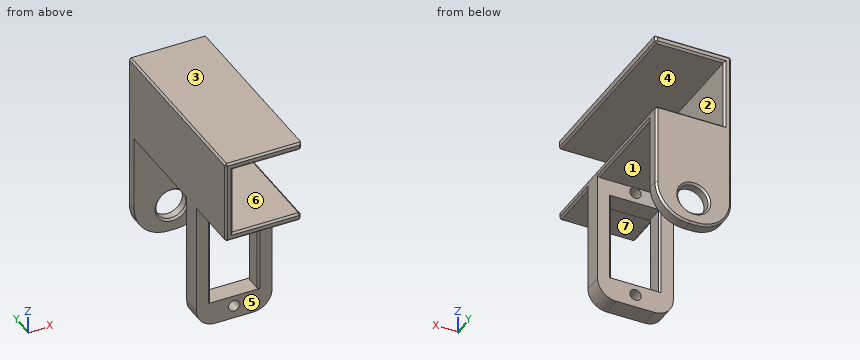
from build123d import *

# Parameters (mm, degrees)
SKETCH1_W           = 20
SKETCH1_H           = 50
BOSS_EXTRUDE1_DEPTH = 2
BOSS_EXTRUDE2_DEPTH = 50
SKETCH3_R           = 4
BOSS_EXTRUDE3_DEPTH = 3
SKETCH4_W           = 12.6
SKETCH4_H           = 23.6
BOSS_EXTRUDE4_DEPTH = 5
CHAMFER1_SIZE       = 0.5
CHAMFER2_SIZE       = 0.5
SKETCH5_R           = 1.5
CUT_EXTRUDE1_DEPTH  = 5


with BuildPart() as part:
    # Sketch1 → Boss-Extrude1 (new body)
    with BuildSketch(Plane.XY):
        with Locations((0, 25)):
            Rectangle(SKETCH1_W, SKETCH1_H)
    extrude(amount=BOSS_EXTRUDE1_DEPTH)

    # Sketch2 → Boss-Extrude2 (add)
    with BuildSketch(Plane.XZ):
        Polygon((-10, 2), (-10, 22.1), (10.1, 22.1), (10.1, 20.1), (-8, 20.1), (-8, 2), align=None)
    extrude(amount=-BOSS_EXTRUDE2_DEPTH)

    # Sketch3 → Boss-Extrude3 (add)
    with BuildSketch(Plane(origin=(0, 50, 0), x_dir=(1, 0, 0), z_dir=(0, 1, 0))):
        with BuildLine():
            Line((1, 28.638755942), (-1, 28.638755942))
            ThreePointArc((-1, 28.638755942), (-7.363961031, 26.002716972), (-10, 19.638755942))
            Line((-10, 19.638755942), (-10, 0))
            Line((-10, 0), (10, 0))
            Line((10, 0), (10, 19.638755942))
            ThreePointArc((10, 19.638755942), (7.363961031, 26.002716972), (1, 28.638755942))
        make_face()
        with Locations(Location((0, 21.5, 0), (0, 0, 270))):
            Circle(SKETCH3_R, mode=Mode.SUBTRACT)
    extrude(amount=-BOSS_EXTRUDE3_DEPTH)

    # Sketch4 → Boss-Extrude4 (add)
    with BuildSketch(Plane(origin=(0, 20, 0), x_dir=(-1, 0, 0), z_dir=(0, -1, 0))):
        with BuildLine():
            Line((-10, 0), (10, 0))
            Line((10, 0), (10, 29))
            ThreePointArc((10, 29), (8.535533906, 32.535533906), (5, 34))
            Line((5, 34), (-5, 34))
            ThreePointArc((-5, 34), (-8.535533906, 32.535533906), (-10, 29))
            Line((-10, 29), (-10, 0))
        make_face()
        with Locations((0, 16)):
            Rectangle(SKETCH4_W, SKETCH4_H, mode=Mode.SUBTRACT)
    extrude(amount=BOSS_EXTRUDE4_DEPTH)

    # Chamfer1
    chamfer1_edges = [part.edges().sort_by_distance(p)[0] for p in [
        (1, 0, 2),
        (-10, 25, 22.1),
        (10.1, 25, 20.1),
        (-8, 0, 11.05),
        (1.05, 0, 20.1),
        (10.1, 0, 21.1),
        (0.05, 0, 22.1),
        (0.05, 50, 22.1),
        (10.1, 50, 21.1),
        (1.05, 50, 20.1),
        (-8, 50, 11.05),
        (-10, 33.5, 0),
        (0, 50, -25.5),
        (0, 50, -28.638755942),
        (-7.363961031, 50, -26.002716972),
        (7.363961031, 50, -26.002716972),
        (10, 25, 2),
        (0, 0, 0),
        (-10, 7.5, 0),
        (10, 33.5, 0),
        (6.3, 20, -16),
        (-6.3, 20, -16),
        (6.3, 15, -16),
        (10, 7.5, 0),
        (-6.3, 15, -16),
        (1, 50, 2),
        (10, 0, 1),
        (-10, 0, 11.05),
        (-10, 50, 1.230622029),
        (10, 50, -8.819377971),
    ]]
    chamfer(chamfer1_edges, length=CHAMFER1_SIZE)

    # Chamfer2
    chamfer2_edges = [part.edges().sort_by_distance(p)[0] for p in [
        (0, 47, -25.5),
    ]]
    chamfer(chamfer2_edges, length=CHAMFER2_SIZE)

    # Sketch5 → Cut-Extrude1 (cut)
    with BuildSketch(Plane(origin=(0, 20, 0), x_dir=(1, 0, 0), z_dir=(0, 1, 0))):
        with Locations(Location((0, 30.585786438, 0), (0, 0, 180))):
            Circle(SKETCH5_R)
        with Locations(Location((0, 1.414213562, 0), (0, 0, 250.528779366))):
            Circle(SKETCH5_R)
    extrude(amount=-CUT_EXTRUDE1_DEPTH, mode=Mode.SUBTRACT)


solid = part.part
Work out the finished part from the listing and answer in its coordinate system (mm). Face numbers are marked on the shaded views. A direction names the side the tool comes from. Round coordinates to 2 decimals unless told otherwise and drop trailing zeros. Write each loop counter-clockwise with the first axis right and the second up, starting at its lowest first coordinate (ties: lowest second). Pieces come first, ordered by that corner, then holes. Notation, with made-up numbers: (-27, -34.75) - (20, -34.75) arc R27 cw to (20, -7.75) - close; hole circle Ø10 at (45.25, 50.5). An arc over 180 degrees is marked (long way). Answer in a Markdown table with one row per item. Add a question column.
1. Given pin 1 (2 mm diameter, centred on y = 17, z = -14.5, fed in from +X); pin 2 (10 mm diameter, centred on x = 1.5, z = 15, fed in from -Y); pin 3 (5 mm diameter, centred on x = 0, z = -30.59, fed in from -Y); pin 4 (11.5 mm diameter, centred on x = -1, y = 5.5, fed in from -Z), each flat-ended and moving along its own axis, determine where each tip first touches the part or whether it passes through.
2. A cutting plane is placed at A-A, the plane y = 21. Determine the outline of the cut face in (x, z), and give its area (3 significant figures).
3. For the marked faces 1, 2 and 3, determine the directions among +Z, -Z, +X, -X, +Y, -Y from which every point of the face is accessible in a straight line to the end or side of a thin tool.
4. A cutting plane is placed at B-B, the plane z = 15.5. Determine the outline of the cut face in (x, y), and give its area (3 significant figures).
5. Find the intervals of material crossed by line 1 along Z through (x, y) = (0, 18.85); line 2 along Z through (x, y) = (1.5, 5); line 3 along X through (y, z) = (17.5, -21), in increasing order. Write a range as from..to.
6. A cutting plane is placed at C-C, the plane z = -21.5. Count the separate pieces of the cut face and the enclosed holes in it, and give its area (3 significant figures).
7. The mould has two halves that part along Z. Classify the marked faces 4, 5, 6 and 7: +Z half, -Z half, draft (parallel to the pull), parting line (faces both ways), or undercut.
Worked out:
| question | item | result |
|---|---|---|
| 1 | pin 1 | x = 10 |
| 1 | pin 2 | through |
| 1 | pin 3 | y = 15 |
| 1 | pin 4 | z = 0 |
| 2 | outline | (-10, 0.5) - (-9.5, 0) - (9.5, 0) - (10, 0.5) - (10, 1.5) - (9.5, 2) - (-8, 2) - (-8, 20.1) - (9.6, 20.1) - (10.1, 20.6) - (10.1, 22.1) - (-9.5, 22.1) - (-10, 21.6) - close |
| 2 | area | 116 mm^2 |
| 3 | face 1 | -Z, +X, -X |
| 3 | face 2 | +X, +Y, -Y |
| 3 | face 3 | +Z, +X, -X, +Y, -Y |
| 4 | outline | (-10, 0.5) - (-9.5, 0) - (-8.5, 0) - (-8, 0.5) - (-8, 49.5) - (-8.5, 50) - (-9.5, 50) - (-10, 49.5) - close |
| 4 | area | 99.5 mm^2 |
| 5 | line 1 | -34..-32.09, -29.09..-27.8, -4.2..-2.91, 0.09..2, 20.1..22.1 |
| 5 | line 2 | 0..2, 20.1..22.1 |
| 5 | line 3 | -10..-6.3, 6.3..10 |
| 6 | separate pieces | 4 |
| 6 | enclosed holes | 0 |
| 6 | area | 70.6 mm^2 |
| 7 | face 4 | undercut |
| 7 | face 5 | draft |
| 7 | face 6 | undercut |
| 7 | face 7 | -Z half |
